from build123d import *

# Parameters (mm, degrees)
CROQUIS1_W              = 30
CROQUIS1_H              = 25.5
SALIENTE_EXTRUIR1_DEPTH = 5
SALIENTE_EXTRUIR2_DEPTH = 25.5
CROQUIS3_R              = 3.5
SALIENTE_EXTRUIR3_DEPTH = 25.5
CROQUIS4_R              = 1.5
CORTAR_EXTRUIR1_DEPTH   = 31
CORTAR_EXTRUIR2_DEPTH   = 31
CORTAR_EXTRUIR3_DEPTH   = 12


with BuildPart() as part:
    # Croquis1 → Saliente-Extruir1 (new body)
    with BuildSketch(Plane(origin=(0, 0, 0), x_dir=(1, 0, 0), z_dir=(0, 1, 0))):
        with Locations((15, 12.75)):
            Rectangle(CROQUIS1_W, CROQUIS1_H)
    extrude(amount=SALIENTE_EXTRUIR1_DEPTH)

    # Croquis2 → Saliente-Extruir2 (add)
    with BuildSketch(Plane.XY):
        Polygon((26.173467515, 5), (30, 8.826532485), (60, 8.826532485), (60, 3.829826023), (30, 3.829826023), (30, 5), align=None)
    extrude(amount=-SALIENTE_EXTRUIR2_DEPTH)

    # Croquis3 → Saliente-Extruir3 (add)
    with BuildSketch(Plane.XY):
        with Locations((2.449489743, 2.5)):
            Circle(CROQUIS3_R)
    extrude(amount=-SALIENTE_EXTRUIR3_DEPTH)

    # Croquis4 → Cortar-Extruir1 (cut)
    with BuildSketch(Plane.XY):
        with Locations((2.449489743, 2.5)):
            Circle(CROQUIS4_R)
    extrude(amount=-CORTAR_EXTRUIR1_DEPTH, mode=Mode.SUBTRACT)

    # Croquis5 → Cortar-Extruir2 (cut)
    with BuildSketch(Plane.XZ.offset(-3.829826023)):
        with BuildLine():
            Line((52.938565695, -10.25), (36.938565695, -10.25))
            ThreePointArc((36.938565695, -10.25), (35.524352133, -10.835786438), (34.938565695, -12.25))
            Line((34.938565695, -12.25), (34.938565695, -13.25))
            ThreePointArc((34.938565695, -13.25), (35.524352133, -14.664213562), (36.938565695, -15.25))
            Line((36.938565695, -15.25), (52.938565695, -15.25))
            ThreePointArc((52.938565695, -15.25), (54.352779258, -14.664213562), (54.938565695, -13.25))
            Line((54.938565695, -13.25), (54.938565695, -12.25))
            ThreePointArc((54.938565695, -12.25), (54.352779258, -10.835786438), (52.938565695, -10.25))
        make_face()
    extrude(amount=-CORTAR_EXTRUIR2_DEPTH, mode=Mode.SUBTRACT)

    # Croquis6 → Cortar-Extruir3 (cut)
    with BuildSketch(Plane.XZ.offset(-3.829826023)):
        with BuildLine():
            Line((36.938565695, -5.25), (30, -5.25))
            Line((30, -5.25), (30, 0))
            Line((30, 0), (60, 0))
            Line((60, 0), (60, -25.5))
            Line((60, -25.5), (30, -25.5))
            Line((30, -25.5), (30, -20.25))
            Line((30, -20.25), (36.938565695, -20.25))
            Line((36.938565695, -20.25), (52.938565695, -20.25))
            ThreePointArc((52.938565695, -20.25), (57.888313164, -18.199747468), (59.938565695, -13.25))
            Line((59.938565695, -13.25), (59.938565695, -12.25))
            ThreePointArc((59.938565695, -12.25), (57.888313164, -7.300252532), (52.938565695, -5.25))
            Line((52.938565695, -5.25), (36.938565695, -5.25))
        make_face()
    extrude(amount=-CORTAR_EXTRUIR3_DEPTH, mode=Mode.SUBTRACT)


solid = part.part
Geometry check sheet. Reference: the model listing, model coordinates, mm. A direction names the side the tool comes from. Round coordinates to 2 decimals unless told otherwise and drop trailing zeros. Order: outer loops, then holes, each group sorted by start corner. A loop starts at its lowest first (then second) coordinate and runs counter-clockwise, first axis right, second up. Notation, with made-up numbers: M 32.25,67 L 58.25,67 A14 cw 58.25,73 Z; hole C 78.5,10.5 d11. An arc over 180 degrees is marked long. Answer in a Markdown table with one row per item. Add a question column.
Item 1: Sectioned sample at A-A, the plane x = 39. Enter the section's corners in (y, z).
Item 2: Draft check along X on faces 5 (the face through (42, 6, -5.25)), 6 (the face through (57.834, 6.293, -18.254)), 7 (the face through (35.51, 6.29, -14.65)). Enter one of: released by +X, released by -X, zero draft, split by the parting line, or undercut.
Item 3: Sectioned sample at C-C, the plane y = 8. Enter the section's corners in (x, z), plus the area to 3 significant figures.
Item 4: Sectioned sample at B-B, the plane y = 2.5. Enter the section's corners in (x, z), plus the area to 3 significant figures.
Item 5: Depth check by flat-ended pin: pin 1 Ø1.5 at (x, y) = (45, 7) entering from -Z; pin 2 Ø5 at (x, z) = (39.5, -11.5) entering from +Y; pin 3 Ø4 at (x, y) = (48.5, 7) entering from +Z; pin 4 Ø2.5 at (y, z) = (4, -17.5) entering from +X. Enter the tip coordinate at first touch or a pass-through.
Item 6: Material ranges on L1, parallel to Z at x = 43, y = 7.25; L2, parallel to Y at x = 5.5, z = -0.75; L3, parallel to Y at x = 31, z = -18.5, recorded low to high. Write a range as [from, to].
Item 7: Sectioned sample at D-D, the plane z = -16. Enter the section's corners in (x, y), plus the area to 3 significant figures.
Item 8: Set-up check for faces 1 (the face through (41, 6, -20.25)), 2 (the face through (17, 0, -13)), 3 (the face through (54.337, 6.293, -14.68)), 4 (the face through (28.06, 6.886, -12.572)): record each of +Z, -Z, +X, -X, +Y, -Y from which the full face is reachable in a straight line by a thin tool's end or side.
Filled in:
| question | item | result |
|---|---|---|
| 1 | outline | M 3.83,-20.25 L 8.83,-20.25 L 8.83,-15.25 L 3.83,-15.25 Z; M 3.83,-10.25 L 8.83,-10.25 L 8.83,-5.25 L 3.83,-5.25 Z |
| 2 | face 5 | zero draft |
| 2 | face 6 | released by +X |
| 2 | face 7 | undercut |
| 3 | outline | M 29.17,-25.5 L 30,-25.5 L 30,-20.25 L 52.94,-20.25 A7 ccw 59.94,-13.25 L 59.94,-12.25 A7 ccw 52.94,-5.25 L 30,-5.25 L 30,0 L 29.17,0 Z; hole M 34.94,-13.25 A2 ccw 36.94,-15.25 L 52.94,-15.25 A2 ccw 54.94,-13.25 L 54.94,-12.25 A2 ccw 52.94,-10.25 L 36.94,-10.25 A2 ccw 34.94,-12.25 Z |
| 3 | area | 353 mm² |
| 4 | outline | M -1.05,-25.5 L 0.95,-25.5 L 0.95,0 L -1.05,0 Z; M 3.95,-25.5 L 30,-25.5 L 30,0 L 3.95,0 Z |
| 4 | area | 715 mm² |
| 5 | pin 1 | stops at z = -20.25 |
| 5 | pin 2 | stops at y = 8.83 |
| 5 | pin 3 | stops at z = -5.25 |
| 5 | pin 4 | stops at x = 59.26 |
| 6 | L1 | z = [-20.25, -15.25], [-10.25, -5.25] |
| 6 | L2 | y = [0, 5] |
| 6 | L3 | y = [3.83, 8.83] |
| 7 | outline | M 4.9,0 L 30,0 L 30,3.83 L 59.38,3.83 L 59.38,8.83 L 30,8.83 L 26.17,5 L 4.9,5 A3.5 ccw long Z; hole C 2.45,2.5 d3 |
| 7 | area | 307 mm² |
| 8 | face 1 | -Z, +X, +Y, -Y |
| 8 | face 2 | +Z, -Z, +X, -Y |
| 8 | face 3 | +Y, -Y |
| 8 | face 4 | +Z, -Z, +Y |
